```python
from build123d import *

# Parameters (mm, degrees)
EXTRUDE_1_DEPTH     = 2
SKETCH_2_R          = 2.25
EXTRUDE_2_DEPTH     = 3
SKETCH_3_R          = 0.676633681
SKETCH_3_R_2        = 0.750657672
CUT_EXTRUDE_1_DEPTH = 10
FILLET_1_R          = 0.25
FILLET_2_R          = 0.25


with BuildPart() as part:
    # 草图1 → 凸台-拉伸1 (new body)
    with BuildSketch(Plane(origin=(0, 0, 0), x_dir=(1, 0, 0), z_dir=(0, 1, 0))):
        with BuildLine():
            Line((5, 0), (14.310335592, 0))
            Line((14.310335592, 0), (14.310335592, 12.5))
            Line((14.310335592, 12.5), (5, 12.5))
            ThreePointArc((5, 12.5), (-1.25, 6.25), (5, 0))
        make_face()
    extrude(amount=EXTRUDE_1_DEPTH)

    # 草图2 → 凸台-拉伸2 (add)
    with BuildSketch(Plane(origin=(0, 2, 0), x_dir=(1, 0, 0), z_dir=(0, 1, 0))):
        with Locations(Location((5, 6.25, 0), (0, 0, 270))):
            Circle(SKETCH_2_R)
    extrude(amount=EXTRUDE_2_DEPTH)

    # 草图3 → 切除-拉伸1 (cut)
    with BuildSketch(Plane(origin=(0, 2, 0), x_dir=(1, 0, 0), z_dir=(0, 1, 0))):
        with Locations(Location((12.810335592, 10, 0), (0, 0, 270))):
            Circle(SKETCH_3_R)
        with Locations(Location((12.810335592, 5, 0), (0, 0, 270))):
            Circle(SKETCH_3_R_2)
    extrude(amount=-CUT_EXTRUDE_1_DEPTH, mode=Mode.SUBTRACT)

    # 圆角1
    fillet_1_edges = [part.edges().sort_by_distance(p)[0] for p in [
        (5, 2, -8.5),
    ]]
    fillet(fillet_1_edges, radius=FILLET_1_R)

    # 圆角2
    fillet_2_edges = [part.edges().sort_by_distance(p)[0] for p in [
        (14.310335592, 1, 0),
        (14.310335592, 1, -12.5),
    ]]
    fillet(fillet_2_edges, radius=FILLET_2_R)


solid = part.part
```
Source: CAD feature listing. Evaluate the final solid. Frame: model axes, mm. A direction names the side the tool comes from. Round coordinates to 2 decimals unless told otherwise and drop trailing zeros. Write each loop counter-clockwise with the first axis right and the second up, starting at its lowest first coordinate (ties: lowest second). Pieces come first, ordered by that corner, then holes. Notation, with made-up numbers: M 68.25,44.25 L 126.25,44.25 A21 cw 126.25,63.25 Z; hole C 5.25,58 d1. An arc over 180 degrees is marked long. Answer as a JSON object with one key per item and string values. Group by question number.
(1) Section query C-C on z = -6.25. Output: boundary loops of the cut face in (x, y).
(2) Reachability of faces 1 (the cylindrical face through (5.676, 3.606, -4.104)), 2 (the flat face through (10, 1, -12.5)) from +Z, -Z, +X, -X, +Y, -Y: full face, straight path, thin tool, end or side. Return the list, or none.
(3) Ray query, line 1 (X direction, y = 0.45, z = -10); line 2 (Z direction, x = 12.25, y = 1.4); line 3 (X direction, y = 1.3, z = -5). Return the intervals inside material, ascending. Write a range as [from, to].
(4) Section query A-A on z = -10. Output: boundary loops of the cut face in (x, y), then the cut area to 3 significant figures.
(5) Section query B-B on x = 13. Output: boundary loops of the cut face in (y, z).
(6) First-contact query: pin 1 (2 mm diameter, centred on x = 12.81, z = -10, fed in from +Y); pin 2 (1 mm diameter, centred on y = 4, z = -7, fed in from +X). Flat tips, straight axial feed; report the tip coordinate or a pass-through.
(7) Mould query, pull axis X, two halves, no side actions, for faces 3 (the flat face through (14.31, 1, -6)), 4 (the cylindrical face through (12.21, 1.01, -9.69)), 5 (the flat face through (9, 1, 0)). Classes: +X half, -X half, draft (parallel to the pull), parting line (faces both ways), or undercut.
(8) Section query D-D on y = 1.7. Output: boundary loops of the cut face in (x, z).
Computed values:
{
 "1": {"outline": "M -1.25,0 L 14.31,0 L 14.31,2 L 7.5,2 A0.25 cw 7.25,2.25 L 7.25,5 L 2.75,5 L 2.75,2.25 A0.25 cw 2.5,2 L -1.25,2 Z"},
 "2": {"face 1": "+Y", "face 2": "-Z, +X, -X, +Y, -Y"},
 "3": {"line 1": "[0, 12.13], [13.49, 14.31]", "line 2": "[-12.5, -10.38], [-9.62, -5.5], [-4.5, 0]", "line 3": "[-1.12, 12.06], [13.56, 14.31]"},
 "4": {"outline": "M 0,0 L 12.13,0 L 12.13,2 L 0,2 Z; M 13.49,0 L 14.31,0 L 14.31,2 L 13.49,2 Z", "area": "25.9 mm^2"},
 "5": {"outline": "M 0,-12.5 L 2,-12.5 L 2,-10.65 L 0,-10.65 Z; M 0,-9.35 L 2,-9.35 L 2,-5.73 L 0,-5.73 Z; M 0,-4.27 L 2,-4.27 L 2,0 L 0,0 Z"},
 "6": {"pin 1": "y = 2", "pin 2": "x = 7.24"},
 "7": {"face 3": "+X half", "face 4": "undercut", "face 5": "draft"},
 "8": {"outline": "M 5,-12.5 L 14.06,-12.5 A0.25 ccw 14.31,-12.25 L 14.31,-0.25 A0.25 ccw 14.06,0 L 5,0 A6.25 ccw Z; hole C 12.81,-5 d1.5; hole C 12.81,-10 d1.35"}
}
